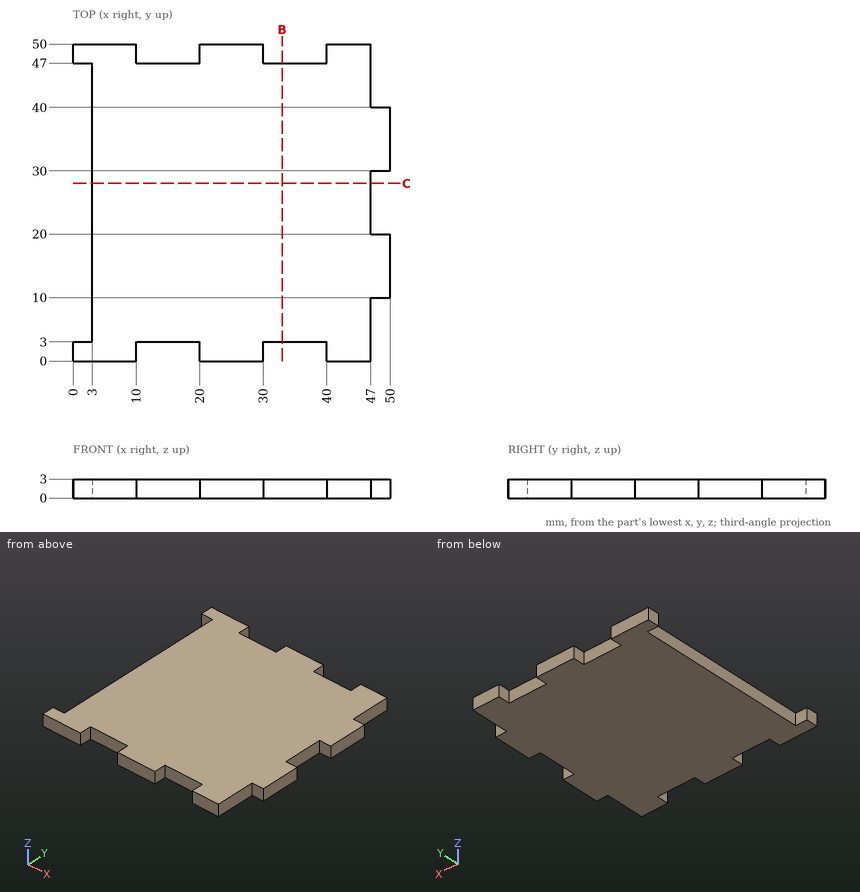
Geometry: see drawing. Coordinates: mm, zero at the bounding-box minimum. Coordinates: 2 decimals unless noted, no trailing zeros. Loops run counter-clockwise (first coordinate to the right, second up) from the corner with the lowest first, then second, coordinate; pieces in that order, holes last.
Q1. Cut plane B-B (x = 33). Output: boundary loops of the cut face in (y, z).
Q2. Contact query for flat-ended pins moving along their axis: pin 1 (1.5 mm diameter, centred on x = 49, z = 1, fed in from +Y); pin 2 (1.5 mm diameter, centred on x = 36.5, z = 2, fed in from -Y); pin 3 (1.5 mm diameter, centred on y = 49, z = 2, fed in from +X); pin 4 (1.5 mm diameter, centred on y = 1, z = 1.5, fed in from -X). Output: stop coordinate, or through.
Q3. Material intervals for line 1 (X direction, y = 27.5, z = 2.05); line 2 (X direction, y = 37.5, z = 1.3), sorted ascending.
Working result:
1. outline: (3, 0) - (47, 0) - (47, 3) - (3, 3) - close
2. pin 1: stops at y = 40
2. pin 2: stops at y = 3
2. pin 3: stops at x = 47
2. pin 4: stops at x = 0
3. line 1: x = 3 to 47
3. line 2: x = 3 to 50
